Here's how the part is built. I have some questions about the finished solid (model axes, mm). A direction names the side the tool comes from. Round coordinates to 2 decimals unless told otherwise and drop trailing zeros. Loops run counter-clockwise (first coordinate to the right, second up) from the corner with the lowest first, then second, coordinate; pieces in that order, holes last. Notation, with made-up numbers: M 67.25,21.25 L 96.25,21.25 A16 ccw 96.25,29.25 Z; hole C -16.5,11 d7. An arc over 180 degrees is marked long. Answer as CSV lines item,"result".
```python
from build123d import *

# Parameters (mm, degrees)
F1_DEPTH = 60
F2_W     = 20
F2_H     = 5
F3_DEPTH = 50
F5_DEPTH = 60.001
F6_W     = 10
F6_H     = 20
F7_DEPTH = 30.001
F8_DEPTH = 5.0010001


with BuildPart() as f1:
    # F0 (on Front) → F1 (new body)
    with BuildSketch(Plane.XZ):
        with BuildLine():
            ThreePointArc((0, 20), (-14.1421356237, 14.1421356237), (-20, 0))
            Line((-20, 0), (0, 0))
            Line((0, 0), (0, 20))
        make_face()
        with BuildLine():
            ThreePointArc((0, 30), (-21.2132034356, 21.2132034356), (-30, 0))
            Line((-30, 0), (-20, 0))
            ThreePointArc((-20, 0), (-14.1421356237, 14.1421356237), (0, 20))
            Line((0, 20), (0, 30))
        make_face()
    extrude(amount=-F1_DEPTH)

    # F2 (on face) → F3 (join)
    with BuildSketch(Plane.YZ):
        with Locations((50, 2.5)):
            Rectangle(F2_W, F2_H)
    extrude(amount=-F3_DEPTH)

    # F0 (on Front) → F5 (cut, through all)
    with BuildSketch(Plane.XZ):
        with BuildLine():
            ThreePointArc((0, 20), (-14.1421356237, 14.1421356237), (-20, 0))
            Line((-20, 0), (0, 0))
            Line((0, 0), (0, 20))
        make_face()
    extrude(amount=-F5_DEPTH, mode=Mode.SUBTRACT)

    # F6 (on Top) → F7 (cut, through all)
    with BuildSketch(Plane.XY):
        with Locations((-5, 10)):
            Rectangle(F6_W, F6_H)
        with BuildLine():
            Line((-10, 20), (0, 20))
            Line((0, 20), (0, 30))
            ThreePointArc((0, 30), (-7.0710678119, 27.0710678119), (-10, 20))
        make_face()
    extrude(amount=F7_DEPTH, mode=Mode.SUBTRACT)

    # F4 (on face) → F8 (cut, through all)
    with BuildSketch(Plane.XY.offset(5)):
        with BuildLine():
            ThreePointArc((-40, 40), (-47.0710678119, 42.9289321881), (-50, 50))
            Line((-50, 50), (-50, 40))
            Line((-50, 40), (-40, 40))
        make_face()
        with BuildLine():
            Line((-40, 60), (-50, 60))
            Line((-50, 60), (-50, 50))
            ThreePointArc((-50, 50), (-47.0710678119, 57.0710678119), (-40, 60))
        make_face()
        with BuildLine():
            Line((-40, 50), (-45, 50))
            ThreePointArc((-45, 50), (-43.5355339059, 46.4644660941), (-40, 45))
            Line((-40, 45), (-40, 50))
        make_face()
        with BuildLine():
            Line((-35, 50), (-40, 50))
            Line((-40, 50), (-40, 45))
            ThreePointArc((-40, 45), (-36.4644660941, 46.4644660941), (-35, 50))
        make_face()
        with BuildLine():
            ThreePointArc((-35, 50), (-36.4644660941, 53.5355339059), (-40, 55))
            Line((-40, 55), (-40, 50))
            Line((-40, 50), (-35, 50))
        make_face()
        with BuildLine():
            ThreePointArc((-40, 55), (-43.5355339059, 53.5355339059), (-45, 50))
            Line((-45, 50), (-40, 50))
            Line((-40, 50), (-40, 55))
        make_face()
    extrude(amount=-F8_DEPTH, mode=Mode.SUBTRACT)

    # F9: F1 across plane


with BuildPart() as f1_1:
    add(f1.part)
    add(f1.part.mirror(Plane.YZ))


solid = f1_1.part
```
1. I want a section at B-B, the plane y = 26. Please give me the cut outline in (x, z), and give its area (3 significant figures).
Evaluation:
outline,"M -30,0 L -20,0 A20 cw -8,18.33 L -8,28.91 A30 ccw Z; M 8,18.33 A20 cw 20,0 L 30,0 A30 ccw 8,28.91 Z"
area,"622 mm²"
2. I want a section at A-A, the plane y = 42. Please give me the cut outline in (x, z), and give its area (3 significant figures).
Evaluation:
outline,"M -46,0 L -20,0 A20 cw 20,0 L 46,0 L 46,5 L 29.58,5 A30 ccw -29.58,5 L -46,5 Z"
area,"947 mm²"
3. If I drill on line 1 (X direction, y = 22.5, z = 14); line 2 (X direction, y = 42.5, z = 14.5); line 3 (Y direction, x = -30.5, z = 4), over which ranges is the centre line in solid material (lowest first)? Write a range as [from, to].
Evaluation:
line 1,"x = [-26.53, -14.28], [14.28, 26.53]"
line 2,"x = [-26.26, -13.77], [13.77, 26.26]"
line 3,"y = [40, 60]"
4. I want a section at C-C, the plane z = 23. Please give me the cut outline in (x, y).
Evaluation:
outline,"M -19.26,0 L -10,0 L -10,20 A10 cw 10,20 L 10,0 L 19.26,0 L 19.26,60 L -19.26,60 Z"
5. Which directions (+Z, -Z, +X, -X, +Y, -Y) give clear straight access to the entire face, cutting with the end or side of a thin tool? Please do faces 1 (the flat face through (-10, 10, 23)), 2 (the flat face through (35, 48, 5)), 3 (the flat face through (-3, 60, 21)), 4 (the flat face through (29, 36, 0)), 5 (the flat face through (-35, 48, 5)).
Evaluation:
face 1,"+Z, -Z, -Y"
face 2,"+Z, +X, +Y, -Y"
face 3,"+Z, -Z, +X, -X, +Y"
face 4,"-Z, +X, -X, +Y, -Y"
face 5,"+Z, -X, +Y, -Y"
6. For P1, Ø2.5, axis at x = 37, z = 1.5, coming from the -Y side; P2, Ø2, axis at x = -25, y = 45, coming from the +Z side; P3, Ø10, axis at x = -36.5, y = 46.5, coming from the +Z side; P4, Ø3, axis at x = -5, y = 24.5, coming from the +Z side, each with a flat end and sliding along its axis, tell me the tip position at first contact or that it passes through.
Evaluation:
P1,"stops at y = 40"
P2,"stops at z = 18"
P3,"stops at z = 5"
P4,"passes through"
7. I want a section at D-D, the plane y = 33. Please give me the cut outline in (x, z).
Evaluation:
outline,"M -30,0 L -20,0 A20 cw 20,0 L 30,0 A30 ccw Z"
